from build123d import *

# Parameters (mm, degrees)
F0_R     = 290
F0_R_2   = 40
F0_R_3   = 4.5
F1_DEPTH = 12
F2_DEPTH = 25
F3_R     = 7
F4_DEPTH = 8


with BuildPart() as f1:
    # F0 (on Top) → F1 (new body)
    with BuildSketch(Plane.XY):
        Circle(F0_R)
        with BuildLine():
            Line((-235, 15), (-115, 15))
            ThreePointArc((-115, 15), (-99.948323, 1.146943), (-112.507639, -15))
            Line((-112.507639, -15), (-232.507639, -15))
            ThreePointArc((-232.507639, -15), (-250.051677, -1.354005), (-235, 15))
        make_face(mode=Mode.SUBTRACT)
        with Locations((-130, -130)):
            Circle(F0_R_2, mode=Mode.SUBTRACT)
        with Locations((-28, -28)):
            Circle(F0_R_3, mode=Mode.SUBTRACT)
        with BuildLine():
            Line((-15, -235), (-15, -115))
            ThreePointArc((-15, -115), (-1.146943, -99.948323), (15, -112.507639))
            Line((15, -112.507639), (15, -232.507639))
            ThreePointArc((15, -232.507639), (1.354005, -250.051677), (-15, -235))
        make_face(mode=Mode.SUBTRACT)
        with Locations((130, -130)):
            Circle(F0_R_2, mode=Mode.SUBTRACT)
        with Locations((28, -28)):
            Circle(F0_R_3, mode=Mode.SUBTRACT)
        with Locations((-28, 28)):
            Circle(F0_R_3, mode=Mode.SUBTRACT)
        with Locations((-130, 130)):
            Circle(F0_R_2, mode=Mode.SUBTRACT)
        with BuildLine():
            Line((15, 235), (15, 115))
            ThreePointArc((15, 115), (1.146943, 99.948323), (-15, 112.507639))
            Line((-15, 112.507639), (-15, 232.507639))
            ThreePointArc((-15, 232.507639), (-1.354005, 250.051677), (15, 235))
        make_face(mode=Mode.SUBTRACT)
        with Locations((28, 28)):
            Circle(F0_R_3, mode=Mode.SUBTRACT)
        with Locations((130, 130)):
            Circle(F0_R_2, mode=Mode.SUBTRACT)
        with BuildLine():
            Line((235, -15), (115, -15))
            ThreePointArc((115, -15), (99.948323, -1.146943), (112.507639, 15))
            Line((112.507639, 15), (232.507639, 15))
            ThreePointArc((232.507639, 15), (250.051677, 1.354005), (235, -15))
        make_face(mode=Mode.SUBTRACT)
    extrude(amount=F1_DEPTH)

    # F0 (on Top) → F2 (cut)
    with BuildSketch(Plane.XY):
        Circle(F0_R)
        with BuildLine():
            Line((-235, 15), (-115, 15))
            ThreePointArc((-115, 15), (-99.948323, 1.146943), (-112.507639, -15))
            Line((-112.507639, -15), (-232.507639, -15))
            ThreePointArc((-232.507639, -15), (-250.051677, -1.354005), (-235, 15))
        make_face(mode=Mode.SUBTRACT)
        with Locations((-130, -130)):
            Circle(F0_R_2, mode=Mode.SUBTRACT)
        with Locations((-28, -28)):
            Circle(F0_R_3, mode=Mode.SUBTRACT)
        with BuildLine():
            Line((-15, -235), (-15, -115))
            ThreePointArc((-15, -115), (-1.146943, -99.948323), (15, -112.507639))
            Line((15, -112.507639), (15, -232.507639))
            ThreePointArc((15, -232.507639), (1.354005, -250.051677), (-15, -235))
        make_face(mode=Mode.SUBTRACT)
        with Locations((130, -130)):
            Circle(F0_R_2, mode=Mode.SUBTRACT)
        with Locations((28, -28)):
            Circle(F0_R_3, mode=Mode.SUBTRACT)
        with Locations((-28, 28)):
            Circle(F0_R_3, mode=Mode.SUBTRACT)
        with Locations((-130, 130)):
            Circle(F0_R_2, mode=Mode.SUBTRACT)
        with BuildLine():
            Line((15, 235), (15, 115))
            ThreePointArc((15, 115), (1.146943, 99.948323), (-15, 112.507639))
            Line((-15, 112.507639), (-15, 232.507639))
            ThreePointArc((-15, 232.507639), (-1.354005, 250.051677), (15, 235))
        make_face(mode=Mode.SUBTRACT)
        with Locations((28, 28)):
            Circle(F0_R_3, mode=Mode.SUBTRACT)
        with Locations((130, 130)):
            Circle(F0_R_2, mode=Mode.SUBTRACT)
        with BuildLine():
            Line((235, -15), (115, -15))
            ThreePointArc((115, -15), (99.948323, -1.146943), (112.507639, 15))
            Line((112.507639, 15), (232.507639, 15))
            ThreePointArc((232.507639, 15), (250.051677, 1.354005), (235, -15))
        make_face(mode=Mode.SUBTRACT)
    extrude(amount=-F2_DEPTH, mode=Mode.SUBTRACT)

    # F3 (on face) → F4 (cut)
    with BuildSketch(Plane.XY.offset(12)):
        with Locations((-28, 28)):
            Circle(F3_R)
        with Locations((28, 28)):
            Circle(F3_R)
        with Locations((-28, -28)):
            Circle(F3_R)
        with Locations((28, -28)):
            Circle(F3_R)
    extrude(amount=-F4_DEPTH, mode=Mode.SUBTRACT)


solid = f1.part
Here's how the part is built. I have some questions about the finished solid (model axes, mm). A direction names the side the tool comes from. Round coordinates to 2 decimals unless told otherwise and drop trailing zeros. Write each loop counter-clockwise with the first axis right and the second up, starting at its lowest first coordinate (ties: lowest second). Pieces come first, ordered by that corner, then holes.
1. I need wall thicknesses on L1, parallel to Y at x = 28, z = 2.5; L2, parallel to Y at x = 28, z = 6.25; L3, parallel to Y at x = -130, z = 9.5. Which ranges of each line are inside material? Lowest first, please.
2. For faces 4 (the flat face through (-4, 4, 0)), 5 (the cylindrical face through (-1.7, 250.02, 5.92)), 6 (the cylindrical face through (-24.77, 21.79, 8.06)), which set-ups out of +Z, -Z, +X, -X, +Y, -Y let a thin tool reach every point of the face, with its end or its side?
3. Will these pins go through, and if not, where does the flat tip stop? pin 1 Ø1.5 at (y, z) = (202.5, 5.5) entering from +X; pin 2 Ø3.5 at (x, z) = (-204.5, 4) entering from -Y; pin 3 Ø7 at (x, y) = (-28, 28) entering from +Z; pin 4 Ø6 at (x, z) = (190, 3) entering from +Y.
4. Suppose I cut it at C-C (x = 0). List the corners of the cut face in (y, z) for me.
5. Suppose I cut it at B-B (y = -130). List the corners of the cut face in (x, z) for me.
6. Suppose I cut it at D-D (x = 129). List the corners of the cut face in (y, z) for me.
7. Suppose I cut it at A-A (z = 6.5). State how many separate pieces and enclosed holes the cut face has, and give its area (3 significant figures).
8. If we mould it in two halves opening along X, with no side actions, what happens to faces 1 (the cylindrical face through (276.608, 87.108, 5.916)), 2 (the flat face through (-4, 4, 12)), 3 (the cylindrical face through (148.458, -165.487, 5.916))? For each: released by +X, released by -X, zero draft, split by the parting line, or undercut.
Answer sheet:
1. L1: y = -288.65 to -32.5, -23.5 to 23.5, 32.5 to 288.65
1. L2: y = -288.65 to -35, -21 to 21, 35 to 288.65
1. L3: y = -259.23 to -170, -90 to -15, 15 to 90, 170 to 259.23
2. face 4: -Z, +X, -X, +Y, -Y
2. face 5: +Z, -Z
2. face 6: +Z
3. pin 1: stops at x = 208.32
3. pin 2: stops at y = -207.35
3. pin 3: passes through
3. pin 4: stops at y = 221.66
4. outline: (-290, 0) - (-250.1, 0) - (-250.1, 12) - (-290, 12) - close; (-99.9, 0) - (99.9, 0) - (99.9, 12) - (-99.9, 12) - close; (250.1, 0) - (290, 0) - (290, 12) - (250.1, 12) - close
5. outline: (-259.23, 0) - (-170, 0) - (-170, 12) - (-259.23, 12) - close; (-90, 0) - (-15, 0) - (-15, 12) - (-90, 12) - close; (15, 0) - (90, 0) - (90, 12) - (15, 12) - close; (170, 0) - (259.23, 0) - (259.23, 12) - (170, 12) - close
6. outline: (-259.73, 0) - (-169.99, 0) - (-169.99, 12) - (-259.73, 12) - close; (-90.01, 0) - (-15, 0) - (-15, 12) - (-90.01, 12) - close; (15, 0) - (90.01, 0) - (90.01, 12) - (15, 12) - close; (169.99, 0) - (259.73, 0) - (259.73, 12) - (169.99, 12) - close
7. separate pieces: 1
7. enclosed holes: 12
7. area: 226,000 mm2
8. face 1: split by the parting line
8. face 2: zero draft
8. face 3: undercut
